Build history of the part. All positions in model axes, mm. Face numbers are marked on the shaded views. A direction names the side the tool comes from. Coordinates: 2 decimals unless noted, no trailing zeros. Loops run counter-clockwise (first coordinate to the right, second up) from the corner with the lowest first, then second, coordinate; pieces in that order, holes last. Notation, with made-up numbers: (55, 33.5) -> (75, 33.5) arc R24 cw to (75, 48.5) -> close; hole circle Ø11 at (-27.75, 9.25). An arc over 180 degrees is marked (long way). One line per item, written item: value. Start each with the question number.
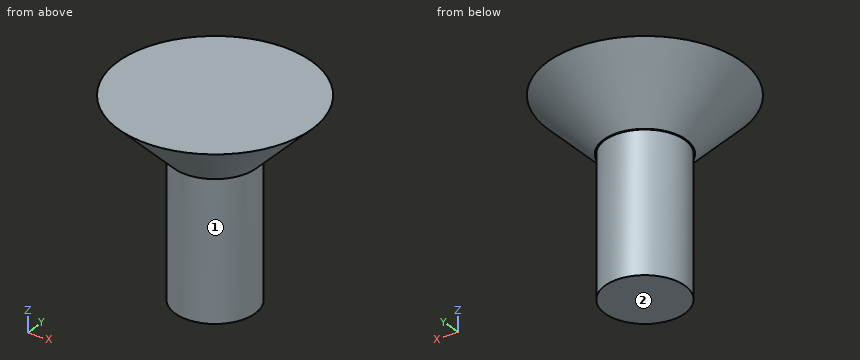
Autodesk Inventor part; units mm, degrees
ref_plane "YZ Plane" through (0, 0, 0) normal (1, 0, 0) x (0, 1, 0)
ref_plane "XZ Plane" through (0, 0, 0) normal (0, 1, 0) x (-1, 0, 0)
ref_plane "XY Plane" through (0, 0, 0) normal (0, 0, 1) x (1, 0, 0)
sketch "スケッチ1" plane through (0, 0, 0) normal (0, 0, 1) x (1, 0, 0)
  circle A0 centre (0, 0) radius 1.65
  dimension "d0" = 3.3
extrude "押し出し1" add sketch "スケッチ1" along normal blind 8
sketch "スケッチ2" plane through (0, 0, 8) normal (0, 0, 1) x (1, 0, 0)
  circle A0 centre (0, 0) radius 4
  dimension "d3" = 8
extrude "押し出し2" add sketch "スケッチ2" against normal blind 2.3
chamfer "面取り1" distance 2.3 angle 45 1 edges at (-4, 0, 5.7)
thread "ねじ1"
properties part number "ネジ皿m4,08" material "鋼、高強度、低合金"
Item 1: Probe probe 1 along X at (y, z) = (0, 3.5); probe 2 along Z at (x, y) = (-2.5, 2); probe 3 along X at (y, z) = (0.5, 5.75). List the from-to ranges inside material, lowest first.
Item 2: Tool access for the marked faces 1 and 2: list every direction of +Z, -Z, +X, -X, +Y, -Y with a clear straight run to the whole face (end or side of a thin tool).
Item 3: Drop flat-ended pins along their axis: pin 1 Ø2 at (x, z) = (-0.5, 4.5) entering from -Y; pin 2 Ø1.5 at (x, z) = (2, 5) entering from -Y; pin 3 Ø3 at (y, z) = (-1.5, 1.5) entering from -X; pin 4 Ø1 at (y, z) = (-2.5, 2) entering from +X. Give the stop position or say it passes through.
Item 4: Band-saw the part on D-D, the plane z = 6.5. List the corners of the cut face in (x, y), and give its area (3 significant figures).
Item 5: Band-saw the part on C-C, the plane z = 4. List the corners of the cut face in (x, y).
Worked out:
1. probe 1: x = -1.65 to 1.65
1. probe 2: z = 7.2 to 8
1. probe 3: x = -1.68 to 1.68
2. face 1: -Z
2. face 2: -Z, +X, -X, +Y, -Y
3. pin 1: stops at y = -1.65
3. pin 2: stops at y = -1.08
3. pin 3: stops at x = -1.65
3. pin 4: passes through
4. outline: circle Ø5 at (0, 0)
4. area: 19.6 mm²
5. outline: circle Ø3.3 at (0, 0)
